Here's the drawing with two shaded views (mm, measured from the low corner). I have some questions. Round coordinates to 2 decimals unless told otherwise and drop trailing zeros. Loops run counter-clockwise (first coordinate to the right, second up) from the corner with the lowest first, then second, coordinate; pieces in that order, holes last.
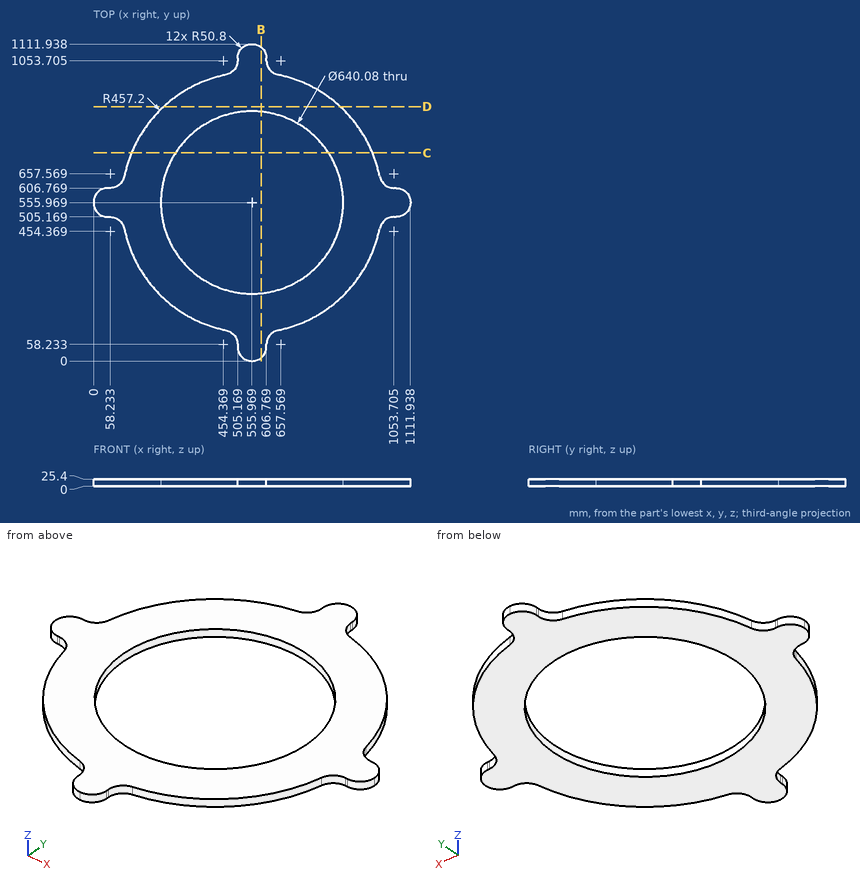
Item 1: Will these pins go through, and if not, where does the flat tip stop? pin 1 (1.5 mm diameter, centred on y = 429.5, z = 20, fed in from -X); pin 2 (3.5 mm diameter, centred on x = 56, z = 18.5, fed in from -Y); pin 3 (4 mm diameter, centred on y = 583.5, z = 11.5, fed in from -X); pin 4 (3 mm diameter, centred on x = 940.5, y = 547, fed in from -Z).
Results list:
pin 1: stops at x = 116.39
pin 2: stops at y = 505.17
pin 3: stops at x = 6.88
pin 4: stops at z = 0
Item 2: If we section it at B-B, the plane x = 588: Please give me the cut outline in (y, z).
Results list:
outline: (11.37, 0) - (237.54, 0) - (237.54, 25.4) - (11.37, 25.4) - close; (874.4, 0) - (1100.57, 0) - (1100.57, 25.4) - (874.4, 25.4) - close
Item 3: If we section it at D-D, the plane y = 892: Please give me the cut outline in (x, z) (1 decimal), then the cut area to 4 significant figures.
Results list:
outline: (245.9, 0) - (866, 0) - (866, 25.4) - (245.9, 25.4) - close
area: 15,750 mm2
Item 4: If I drill on line 1 along Y through (x, z) = (398, 21.75) (1 decimal); line 2 along Y through (x, z) = (745, 11.5); line 3 along X through (y, z) = (531, 20.75) (1 decimal), over which ranges is the centre line in solid material (lowest first)?
Results list:
line 1: y = 126.9 to 277.6, 834.3 to 985
line 2: y = 139.68 to 297.72, 814.22 to 972.26
line 3: x = 6.6 to 236.9, 875 to 1105.4
Item 5: If we section it at C-C, the plane y = 730: Please give me the cut outline in (x, z), then the cut area to 3 significant figures.
Results list:
outline: (133.19, 0) - (287.38, 0) - (287.38, 25.4) - (133.19, 25.4) - close; (824.56, 0) - (978.75, 0) - (978.75, 25.4) - (824.56, 25.4) - close
area: 7,830 mm2
